CAD build for the part. Positions are in the model's coordinates, mm. A direction names the side the tool comes from. Give positions to 0.01 mm unless a question says otherwise; leave off trailing zeros. Loops run counter-clockwise (first coordinate to the right, second up) from the corner with the lowest first, then second, coordinate; pieces in that order, holes last. Notation, with made-up numbers: M 26.5,88 L 54.5,88 A16 ccw 54.5,115 Z; hole C -4,-20.75 d6. An arc over 180 degrees is marked long. Answer as CSV lines item,"result".
```python
from build123d import *

# Parameters (mm, degrees)
SKETCH1_R           = 25
SKETCH1_R_2         = 16
BOSS_EXTRUDE1_DEPTH = 10
SKETCH1_8_R         = 25
SKETCH1_8_R_2       = 16
BOSS_EXTRUDE3_DEPTH = 35
SKETCH1_9_R         = 25
SKETCH1_9_R_2       = 16
BOSS_EXTRUDE4_DEPTH = 48
SKETCH7_R           = 10
BOSS_EXTRUDE5_DEPTH = 10
BOSS_EXTRUDE6_START = 2.5
SKETCH7_5_R         = 19
SKETCH7_5_R_2       = 10
BOSS_EXTRUDE6_DEPTH = 15
FILLET1_R           = 5
FILLET2_R           = 12
FILLET3_R           = 12
FILLET4_R           = 6
FILLET5_START       = 29.9999999
FILLET5_DEPTH       = 15.0000001
FILLET5_START_2     = 35
FILLET5_2_DEPTH     = 10
FILLET5_START_3     = -64
FILLET5_3_DEPTH     = 63.196428571
FILLET6_R           = 6
FILLET7_START       = -45
FILLET7_DEPTH       = 16
FILLET7_START_2     = -88
FILLET7_2_DEPTH     = 87.035714286
FILLET7_3_DEPTH     = 25
FILLET8_R           = 12
FILLET9_R           = 12
FILLET10_R          = 6
FILLET11_R          = 12
FILLET12_R          = 12
FILLET13_R          = 5
FILLET14_R          = 5
SKETCH11_R          = 5
CUT_EXTRUDE1_DEPTH  = 132.658649545


with BuildPart() as part:
    # Sketch1 → Boss-Extrude1 (new body)
    # profile 1 of 3: a face of its own
    with BuildSketch(Plane(origin=(0, 0, 0), x_dir=(1, 0, 0), z_dir=(0, 1, 0))):
        with BuildLine():
            Line((-45, 28), (-45, 0))
            Line((-45, 0), (45, 0))
            Line((45, 0), (45, 28))
            Line((45, 28), (69, 28))
            Line((69, 28), (69, 78))
            Line((69, 78), (45, 78))
            Line((45, 78), (45, 53))
            Line((45, 53), (25, 53))
            Line((25, 53), (25, 28))
            ThreePointArc((25, 28), (0, 3), (-25, 28))
            Line((-25, 28), (-25, 53))
            Line((-25, 53), (-45, 53))
            Line((-45, 53), (-45, 78))
            Line((-45, 78), (-69, 78))
            Line((-69, 78), (-69, 28))
            Line((-69, 28), (-45, 28))
        make_face()
    # profile 2 of 3: a face of its own
    with BuildSketch(Plane(origin=(0, 0, 0), x_dir=(1, 0, 0), z_dir=(0, 1, 0))):
        with Locations((0, 28)):
            Circle(SKETCH1_R)
        with Locations(Location((0, 28, 0), (0, 0, 270))):
            Circle(SKETCH1_R_2, mode=Mode.SUBTRACT)
    # profile 3 of 3: a face of its own
    with BuildSketch(Plane(origin=(0, 0, 0), x_dir=(1, 0, 0), z_dir=(0, 1, 0))):
        with BuildLine():
            Line((-75, 78), (-69, 78))
            Line((-69, 78), (-45, 78))
            Line((-45, 78), (-45, 53))
            Line((-45, 53), (-25, 53))
            Line((-25, 53), (-25, 28))
            ThreePointArc((-25, 28), (0, 53), (25, 28))
            Line((25, 28), (25, 53))
            Line((25, 53), (45, 53))
            Line((45, 53), (45, 78))
            Line((45, 78), (69, 78))
            Line((69, 78), (75, 78))
            Line((75, 78), (75, 88))
            Line((75, 88), (35, 88))
            Line((35, 88), (35, 63))
            Line((35, 63), (0, 63))
            Line((0, 63), (-35, 63))
            Line((-35, 63), (-35, 88))
            Line((-35, 88), (-75, 88))
            Line((-75, 88), (-75, 78))
        make_face()
    extrude(amount=BOSS_EXTRUDE1_DEPTH)

    # Sketch1<8> → Boss-Extrude3 (add)
    # profile 1 of 2: a face of its own
    with BuildSketch(Plane(origin=(0, 0, 0), x_dir=(1, 0, 0), z_dir=(0, 1, 0))):
        with BuildLine():
            Line((-75, 78), (-69, 78))
            Line((-69, 78), (-45, 78))
            Line((-45, 78), (-45, 53))
            Line((-45, 53), (-25, 53))
            Line((-25, 53), (-25, 28))
            ThreePointArc((-25, 28), (0, 53), (25, 28))
            Line((25, 28), (25, 53))
            Line((25, 53), (45, 53))
            Line((45, 53), (45, 78))
            Line((45, 78), (69, 78))
            Line((69, 78), (75, 78))
            Line((75, 78), (75, 88))
            Line((75, 88), (35, 88))
            Line((35, 88), (35, 63))
            Line((35, 63), (0, 63))
            Line((0, 63), (-35, 63))
            Line((-35, 63), (-35, 88))
            Line((-35, 88), (-75, 88))
            Line((-75, 88), (-75, 78))
        make_face()
    # profile 2 of 2: a face of its own
    with BuildSketch(Plane(origin=(0, 0, 0), x_dir=(1, 0, 0), z_dir=(0, 1, 0))):
        with Locations((0, 28)):
            Circle(SKETCH1_8_R)
        with Locations(Location((0, 28, 0), (0, 0, 270))):
            Circle(SKETCH1_8_R_2, mode=Mode.SUBTRACT)
    extrude(amount=BOSS_EXTRUDE3_DEPTH)

    # Sketch1<9> → Boss-Extrude4 (add)
    with BuildSketch(Plane(origin=(0, 0, 0), x_dir=(1, 0, 0), z_dir=(0, 1, 0))):
        with Locations((0, 28)):
            Circle(SKETCH1_9_R)
        with Locations(Location((0, 28, 0), (0, 0, 270))):
            Circle(SKETCH1_9_R_2, mode=Mode.SUBTRACT)
    extrude(amount=BOSS_EXTRUDE4_DEPTH)

    # Sketch7 → Boss-Extrude5 (add)
    with BuildSketch(Plane(origin=(45, 0, 0), x_dir=(0, 0, -1), z_dir=(1, 0, 0))):
        with BuildLine():
            Line((56, 0), (0, 0))
            Line((0, 0), (9, -56))
            ThreePointArc((9, -56), (28, -75), (47, -56))
            Line((47, -56), (56, 0))
        make_face()
        with Locations((28, -56)):
            Circle(SKETCH7_R, mode=Mode.SUBTRACT)
    boss_extrude5 = extrude(amount=-BOSS_EXTRUDE5_DEPTH)

    # Sketch7<5> → Boss-Extrude6 (add)
    with BuildSketch(Plane(origin=(45, 0, 0), x_dir=(0, 0, -1), z_dir=(1, 0, 0)).offset(BOSS_EXTRUDE6_START)):
        with Locations((28, -56)):
            Circle(SKETCH7_5_R)
        with Locations((28, -56)):
            Circle(SKETCH7_5_R_2, mode=Mode.SUBTRACT)
    boss_extrude6 = extrude(amount=-BOSS_EXTRUDE6_DEPTH)

    # Fillet1
    fillet1_edges = [part.edges().sort_by_distance(p)[0] for p in [
        (35, 0, -28),
    ]]
    fillet(fillet1_edges, radius=FILLET1_R)

    # Fillet2
    fillet2_edges = [part.edges().sort_by_distance(p)[0] for p in [
        (45, 5, -28),
    ]]
    fillet(fillet2_edges, radius=FILLET2_R)

    # Fillet3
    fillet3_edges = [part.edges().sort_by_distance(p)[0] for p in [
        (69, 5, -28),
    ]]
    fillet(fillet3_edges, radius=FILLET3_R - 0.0001)  # a hair under: the kernel refuses the full size

    # Fillet4
    fillet4_edges = [part.edges().sort_by_distance(p)[0] for p in [
        (69, 5, -78),
    ]]
    fillet(fillet4_edges, radius=FILLET4_R - 0.0001)  # a hair under: the kernel refuses the full size

    # Fillet5: read off the stored shape, not the designer's step
    # Fillet5 outline → Fillet5 (add)
    with BuildSketch(Plane.YZ.offset(FILLET5_START)):
        with BuildLine():
            ThreePointArc((-21.033047615, -52.619688776), (-11.709098144, -56.128625688), (-4.495715646, -63))
            Line((-4.495715646, -63), (0, -63))
            Line((0, -63), (0, -56))
            Line((0, -56), (-21.033047615, -52.619688776))
        make_face()
    extrude(amount=FILLET5_DEPTH)

    # Fillet5 2 outline → Fillet5 2 (add)
    with BuildSketch(Plane.YZ.offset(FILLET5_START_2)):
        with BuildLine():
            ThreePointArc((-4.495715646, -63), (-1.150397185, -69.806519203), (0, -77.302948058))
            Line((0, -77.302948058), (0, -63))
            Line((0, -63), (-4.495715646, -63))
        make_face()
    extrude(amount=FILLET5_2_DEPTH)

    # Fillet5 3 outline → Fillet5 3 (cut)
    with BuildSketch(Plane.XY.offset(FILLET5_START_3)):
        with BuildLine():
            Line((29.9999999, -23), (35, -23))
            Line((35, -23), (35, -5))
            ThreePointArc((35, -5), (33.535533906, -1.464466094), (30, 0))
            Line((30, 0), (29.9999999, -23))
        make_face()
    extrude(amount=FILLET5_3_DEPTH, mode=Mode.SUBTRACT)

    # Mirror2: Boss-Extrude5, Boss-Extrude6 across plane
    add(boss_extrude5.mirror(Plane(origin=(0, 0, 0), x_dir=(0, 0, 1), z_dir=(1, 0, 0))))
    add(boss_extrude6.mirror(Plane(origin=(0, 0, 0), x_dir=(0, 0, 1), z_dir=(1, 0, 0))))

    # Fillet6
    fillet6_edges = [part.edges().sort_by_distance(p)[0] for p in [
        (-35, 0, -28),
    ]]
    fillet(fillet6_edges, radius=FILLET6_R)

    # Fillet7: read off the stored shape, not the designer's step
    # Fillet7 outline → Fillet7 (add)
    with BuildSketch(Plane.YZ.offset(FILLET7_START)):
        with BuildLine():
            ThreePointArc((-21.033047615, -52.619688776), (-5.971418739, -61.088352929), (0, -77.302948058))
            Line((0, -77.302948058), (0, -56))
            Line((0, -56), (-21.033047615, -52.619688776))
        make_face()
    extrude(amount=FILLET7_DEPTH)

    # Fillet7 2 outline → Fillet7 2 (cut)
    with BuildSketch(Plane.XY.offset(FILLET7_START_2)):
        with BuildLine():
            Line((-29, -23), (-29, 0))
            ThreePointArc((-29, 0), (-33.242640687, -1.757359313), (-35, -6))
            Line((-35, -6), (-35, -23))
            Line((-35, -23), (-29, -23))
        make_face()
    extrude(amount=FILLET7_2_DEPTH, mode=Mode.SUBTRACT)

    # Fillet7 3 outline → Fillet7 3 (cut)
    with BuildSketch(Plane.XY.offset(FILLET7_START_2)):
        with BuildLine():
            Line((-29, 0), (-35, 0))
            Line((-35, 0), (-35, -6))
            ThreePointArc((-35, -6), (-33.242640687, -1.757359313), (-29, 0))
        make_face()
    extrude(amount=FILLET7_3_DEPTH, mode=Mode.SUBTRACT)

    # Fillet8
    fillet8_edges = [part.edges().sort_by_distance(p)[0] for p in [
        (-45, 5, -28),
    ]]
    fillet(fillet8_edges, radius=FILLET8_R)

    # Fillet9
    fillet9_edges = [part.edges().sort_by_distance(p)[0] for p in [
        (-69, 5, -28),
    ]]
    fillet(fillet9_edges, radius=FILLET9_R - 0.0001)  # a hair under: the kernel refuses the full size

    # Fillet10
    fillet10_edges = [part.edges().sort_by_distance(p)[0] for p in [
        (-69, 5, -78),
    ]]
    fillet(fillet10_edges, radius=FILLET10_R - 0.0001)  # a hair under: the kernel refuses the full size

    # Fillet11
    fillet11_edges = [part.edges().sort_by_distance(p)[0] for p in [
        (45, 22.5, -53),
    ]]
    fillet(fillet11_edges, radius=FILLET11_R)

    # Fillet12
    fillet12_edges = [part.edges().sort_by_distance(p)[0] for p in [
        (-45, 22.5, -53),
    ]]
    fillet(fillet12_edges, radius=FILLET12_R)

    # Fillet13
    fillet13_edges = [part.edges().sort_by_distance(p)[0] for p in [
        (45, 22.5, -78),
    ]]
    fillet(fillet13_edges, radius=FILLET13_R)

    # Fillet14
    fillet14_edges = [part.edges().sort_by_distance(p)[0] for p in [
        (-45, 22.5, -78),
    ]]
    fillet(fillet14_edges, radius=FILLET14_R)

    # Sketch11 → Cut-Extrude1 (cut, through all)
    with BuildSketch(Plane.XY.offset(-78)):
        with Locations((63, 23)):
            Circle(SKETCH11_R)
    cut_extrude1 = extrude(amount=-CUT_EXTRUDE1_DEPTH, mode=Mode.SUBTRACT)

    # Mirror8: Cut-Extrude1 across plane
    add(cut_extrude1.mirror(Plane(origin=(0, 0, 0), x_dir=(0, 0, 1), z_dir=(1, 0, 0))), mode=Mode.SUBTRACT)


solid = part.part
```
Q1. Wall check: line 1 (X direction, y = 32, z = -28); line 2 (X direction, y = -49, z = -13); line 3 (Y direction, x = -63, z = -84). Give the ranges that are in metal, low to high. Write a range as [from, to].
Solution:
line 1,"x = [-25, -16], [16, 25]"
line 2,"x = [-47.5, -32.5], [32.5, 47.5]"
line 3,"y = [0, 18], [28, 35]"
Q2. Mould opens along Y. For faces 5 (the cylindrical face through (-39.976, -6.133, -60.901)), 6 (the flat face through (-69, 5, -56)), 7 (the cylindrical face through (40.105, -74.548, -23.881)) say: released by +Y, released by -Y, zero draft, split by the parting line, or undercut.
Solution:
face 5,"released by -Y"
face 6,"zero draft"
face 7,"undercut"
Q3. Cut at B-B (x = 0). Write the cut outline in (y, z).
Solution:
outline,"M 0,-63 L 35,-63 L 35,-53 L 48,-53 L 48,-44 L 0,-44 Z; M 0,-12 L 48,-12 L 48,-3 L 10,-3 L 10,0 L 0,0 Z"
Q4. Cut at A-A (y = 23). Give the number of separate pieces and of enclosed holes in the cut face, and give its area (3 significant figures).
Solution:
separate pieces,"3"
enclosed holes,"1"
area,"3,180 mm²"
Q5. Cut at D-D (y = -29.5). Write the cut outline in (x, z).
Solution:
outline,"M -45,-51.26 L -35,-51.26 L -35,-4.74 L -45,-4.74 Z; M 35,-51.26 L 45,-51.26 L 45,-4.74 L 35,-4.74 Z"
Q6. Pin check, flat tips, straight feed: P1, Ø12, axis at x = -16, y = 25.5, coming from the -Z side; P2, Ø11.5, axis at y = -56, z = -28, coming from the -X side; P3, Ø12, axis at x = 36, y = -17.5, coming from the -Z side; P4, Ø1, axis at y = -27.5, z = -46, coming from the +X side. Stop position of each tip, or through.
Solution:
P1,"stops at z = -63"
P2,"passes through"
P3,"stops at z = -56.26"
P4,"stops at x = 45"
Q7. Which spindle directions (+Z, -Z, +X, -X, +Y, -Y) get a long thin tool onto all of the face, cutting with end or side? Do faces 1 (the flat face through (29, 22, -53)), 2 (the flat face through (35, 15, -75)), 3 (the cylindrical face through (-41.39, 22.68, -56.42)), 4 (the flat face through (0, 0, -46)). Say none if no direction does.
Solution:
face 1,"+Z, +X, +Y"
face 2,"-Z, +Y, -Y"
face 3,"+Z, -X, +Y"
face 4,"+Z, -Z, -Y"
